```python
from build123d import *

# Parameters (mm, degrees)
BOSS_EXTRUDE1_DEPTH = 10
FILLET11_R          = 3


with BuildPart() as part:
    # Sketch2 → Boss-Extrude1 (new body)
    with BuildSketch(Plane.XY):
        Polygon((-60, 9.242640687), (-42, 27.242640687), (-42, 12.242640687), (-27, 27.242640687), (-27, 12.242640687), (-12, 27.242640687), (-12, 12.242640687), (3, 27.242640687), (3, -3), (-123, -3), (-123, 27.242640687), (-108, 12.242640687), (-108, 27.242640687), (-93, 12.242640687), (-93, 27.242640687), (-78, 12.242640687), (-78, 27.242640687), align=None)
        Polygon((-60, 5), (-45, 20), (-45, 5), (-30, 20), (-30, 5), (-15, 20), (-15, 5), (0, 20), (0, 0), (-120, 0), (-120, 20), (-105, 5), (-105, 20), (-90, 5), (-90, 20), (-75, 5), (-75, 20), align=None, mode=Mode.SUBTRACT)
    extrude(amount=BOSS_EXTRUDE1_DEPTH)

    # Fillet11
    fillet11_edges = [part.edges().sort_by_distance(p)[0] for p in [
        (-85.5, 19.742640687, 10),
        (-93, 19.742640687, 10),
        (-100.5, 19.742640687, 10),
        (-108, 19.742640687, 10),
        (-115.5, 19.742640687, 10),
        (-123, 12.121320344, 10),
        (-60, -3, 10),
        (3, 12.121320344, 10),
        (-4.5, 19.742640687, 10),
        (-12, 19.742640687, 10),
        (-69, 18.242640687, 10),
        (-19.5, 19.742640687, 10),
        (-27, 19.742640687, 10),
        (-34.5, 19.742640687, 10),
        (-42, 19.742640687, 10),
        (-51, 18.242640687, 10),
        (-78, 19.742640687, 10),
    ]]
    fillet(fillet11_edges, radius=FILLET11_R - 0.0001)  # a hair under: the kernel refuses the full size


solid = part.part
```
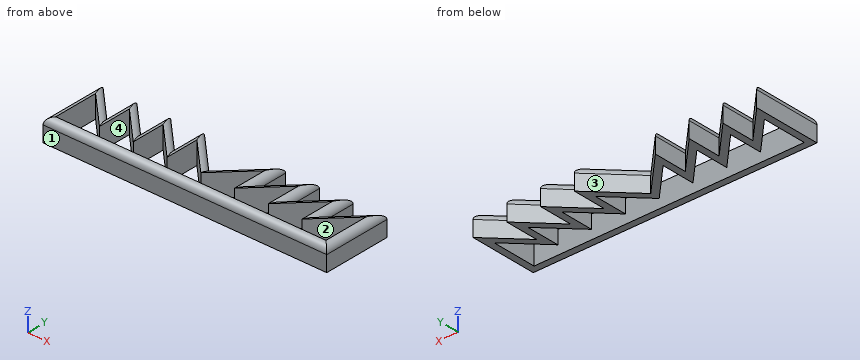
Work out the finished part from the listing and answer in its coordinate system (mm). Face numbers are marked on the shaded views. A direction names the side the tool comes from. Round coordinates to 2 decimals unless told otherwise and drop trailing zeros. Write each question's results on one line, items separated by ' | '.
Q1. Which of the six approach directions +Z, -Z, +X, -X, +Y, -Y give full straight-line access (tool end or side, diameter ignored) to the marked faces 3 and 4?
Data:
face 3: +Z, -Z, +Y | face 4: +Z, -Z
Q2. Determine the mould class of the marked faces 1 and 2 for opening direction X: released by +X, released by -X, zero draft, split by the parting line, or undercut.
Data:
face 1: zero draft | face 2: undercut
Q3. Straight lines are drawn through the part: line 1 along X through (y, z) = (4.5, 4.25); line 2 along Y through (x, z) = (-57, 2.75); line 3 along Y through (x, z) = (-85.5, 9). For each, find the intervals that lie inside material, in ascending order. Write a range as [from, to].
Data:
line 1: [-123, -120], [0, 3] | line 2: [-3, 0], [8, 12.24] | line 3: [-2.24, 0], [15.5, 18.66]
Q4. Section B-B, the plane y = 7.5 is taken. Give the number of separate pieces and of enclosed holes in the cut face, then the cut area to 3 significant figures.
Data:
separate pieces: 9 | enclosed holes: 0 | area: 254 mm^2
Q5. Flat-ended cylindrical pins translate along their axes: P1, Ø5, axis at x = -38.5, z = 8, coming from the +Y side; P2, Ø3, axis at y = 8, z = 8.5, coming from the -X side; P3, Ø4, axis at x = -99, z = 7, coming from the +Y side; P4, Ø1.5, axis at x = -78, z = 3.5, coming from the +Y side. Find the tip coordinate at first contact, or state that the pin passes through.
Data:
P1: y = 18.13 | P2: x = -123 | P3: y = 20.24 | P4: y = 27.24
